Read the model definition and answer for the solid it produces. Units are mm, in the model's axes. A direction names the side the tool comes from. Coordinates: 2 decimals unless noted, no trailing zeros. Write each loop counter-clockwise with the first axis right and the second up, starting at its lowest first coordinate (ties: lowest second). Pieces come first, ordered by that corner, then holes. Notation, with made-up numbers: (26.5, 18) - (65.5, 18) arc R29 cw to (65.5, 51) - close; hole circle Ø7 at (63, 9). An arc over 180 degrees is marked (long way). Return JSON: item names as keys, results as strings.
```python
from build123d import *

# Parameters (mm, degrees)
F1_DEPTH = 10


with BuildPart() as f1:
    # F0 (on Top) → F1 (new body)
    with BuildSketch(Plane.XY):
        with BuildLine():
            Line((50.6, 0), (0, 0))
            Line((0, 0), (-50.6, 0))
            ThreePointArc((-50.6, 0), (-52.367767, 0.732233), (-53.1, 2.5))
            Line((-53.1, 2.5), (-53.1, 14))
            ThreePointArc((-53.1, 14), (-52.367767, 15.767767), (-50.6, 16.5))
            Line((-50.6, 16.5), (-50.35, 16.5))
            ThreePointArc((-50.35, 16.5), (-49.108107, 17.75), (-50.35, 19))
            Line((-50.35, 19), (-53.1, 19))
            ThreePointArc((-53.1, 19), (-54.867767, 18.267767), (-55.6, 16.5))
            Line((-55.6, 16.5), (-55.6, 0))
            ThreePointArc((-55.6, 0), (-54.867767, -1.767767), (-53.1, -2.5))
            Line((-53.1, -2.5), (0, -2.5))
            Line((0, -2.5), (53.1, -2.5))
            ThreePointArc((53.1, -2.5), (54.867767, -1.767767), (55.6, 0))
            Line((55.6, 0), (55.6, 16.5))
            ThreePointArc((55.6, 16.5), (54.867767, 18.267767), (53.1, 19))
            Line((53.1, 19), (50.35, 19))
            ThreePointArc((50.35, 19), (49.1, 17.75), (50.35, 16.5))
            Line((50.35, 16.5), (50.6, 16.5))
            ThreePointArc((50.6, 16.5), (52.367767, 15.767767), (53.1, 14))
            Line((53.1, 14), (53.1, 2.5))
            ThreePointArc((53.1, 2.5), (52.367767, 0.732233), (50.6, 0))
        make_face()
    extrude(amount=F1_DEPTH)


solid = f1.part
```
(1) Straight lines are drawn through the part: line 1 (X direction, y = 8, z = 9.5); line 2 (Y direction, x = 36.5, z = 5.75); line 3 (X direction, y = 1.5, z = 9.75). For each, find the intervals that lie inside material, in ascending order. Write a range as from..to.
Answer:
{"line 1": "-55.6..-53.1, 53.1..55.6", "line 2": "-2.5..0", "line 3": "-55.6..-52.89, 52.89..55.6"}
(2) Which of the six approach directions +Z, -Z, +X, -X, +Y, -Y give full straight-line access (tool end or side, diameter ignored) to faces 1 (the face through (-55.6, 8, 5)), 2 (the face through (-52.348, 0.713, 4.93))?
Answer:
{"face 1": "+Z, -Z, -X, +Y, -Y", "face 2": "+Z, -Z"}
(3) A cutting plane is placed at D-D (y = 1.5). Determine the outline of the cut face in (x, z).
Answer:
{"outline": "(-55.6, 0) - (-52.89, 0) - (-52.89, 10) - (-55.6, 10) - close; (52.89, 0) - (55.6, 0) - (55.6, 10) - (52.89, 10) - close"}
(4) Determine the mould class of faces 3 (the face through (-54.887, -1.748, 4.93)), 4 (the face through (1, 0, 5)), 5 (the face through (-0.3, -0.5, 10)) for opening direction X: +X half, -X half, draft (parallel to the pull), parting line (faces both ways), or undercut.
Answer:
{"face 3": "-X half", "face 4": "undercut", "face 5": "draft"}
(5) A flat-ended cylindrical pin translates along its axis: P1, Ø1.5, axis at x = -41.5, z = 7, coming from the +Y side. Find the tip coordinate at first contact, or state that the pin passes through.
Answer:
{"P1": "y = 0"}
(6) A cutting plane is placed at A-A (y = 10.5). Determine the outline of the cut face in (x, z), and give its area (3 significant figures).
Answer:
{"outline": "(-55.6, 0) - (-53.1, 0) - (-53.1, 10) - (-55.6, 10) - close; (53.1, 0) - (55.6, 0) - (55.6, 10) - (53.1, 10) - close", "area": "50.0 mm²"}
(7) A cutting plane is placed at B-B (z = 9). Determine the outline of the cut face in (x, y).
Answer:
{"outline": "(-55.6, 0) arc R2.5 ccw to (-53.1, -2.5) - (53.1, -2.5) arc R2.5 ccw to (55.6, 0) - (55.6, 16.5) arc R2.5 ccw to (53.1, 19) - (50.35, 19) arc R1.25 ccw to (50.35, 16.5) - (50.6, 16.5) arc R2.5 cw to (53.1, 14) - (53.1, 2.5) arc R2.5 cw to (50.6, 0) - (-50.6, 0) arc R2.5 cw to (-53.1, 2.5) - (-53.1, 14) arc R2.5 cw to (-50.6, 16.5) - (-50.35, 16.5) arc R1.25 ccw to (-50.35, 19) - (-53.1, 19) arc R2.5 ccw to (-55.6, 16.5) - close"}
(8) A cutting plane is placed at C-C (x = -30). Determine the outline of the cut face in (y, z), and give its area (3 significant figures).
Answer:
{"outline": "(-2.5, 0) - (0, 0) - (0, 10) - (-2.5, 10) - close", "area": "25.0 mm²"}
